Geometry: final body of the model. Coordinates: model frame, mm. Face numbers are marked on the shaded views. Give positions to 0.01 mm unless a question says otherwise; leave off trailing zeros. Order: outer loops, then holes, each group sorted by start corner. A loop starts at its lowest first (then second) coordinate and runs counter-clockwise, first axis right, second up. Notation, with made-up numbers: (-17.5, 18.25) -> (-10.5, 18.25) arc R11 cw to (-10.5, 31.25) -> close; hole circle Ø1 at (11.5, -22). An arc over 180 degrees is marked (long way). Answer in a Markdown table with one row per item. Add a question column.
Q1. Cut plane D-D on x = 12. Return the cut outline in (y, z).
Q2. Line query: line 1 along X through (y, z) = (2, 1.75); line 2 along X through (y, z) = (1, 0.5); line 3 along Z through (x, y) = (9, 6.5). Output: solid intervals per line, ascending. Write a range as from..to.
Q3. Cut plane B-B on y = 23. Return the cut outline in (x, z).
Q4. Cut plane A-A on z = 3.75. Return the cut outline in (x, y).
Q5. Contact query for flat-ended pins moving along their axis: P1, Ø3, axis at y = 3, z = 5.5, coming from the -X side; P2, Ø1.5, axis at x = 12, y = 29.5, coming from the -Z side. Output: stop coordinate, or through.
Q6. Cut plane C-C on x = 21. Return the cut outline in (y, z), and give its area (3 significant figures).
Q7. Pull-direction query (X, two-part tool) for the marked faces 1, 2, 3 and 4; classes: +X half, -X half, draft (parallel to the pull), parting line (faces both ways), or undercut.
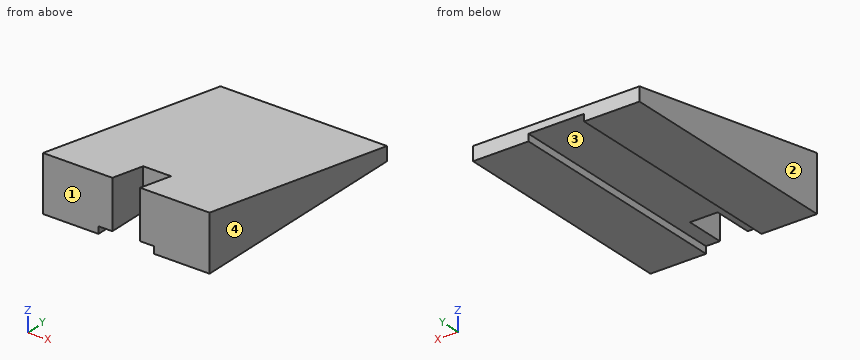
Autodesk Fusion 360 part; units mm, degrees
sketch "Sketch1" plane through (0, 0, 0) normal (0, 0, 1) x (1, 0, 0)
  line L0 (0, 0) -> (24, 0)
  line L1 (24, 0) -> (24, 34)
  line L2 (24, 34) -> (0, 34)
  line L3 (0, 34) -> (0, 0)
  line L4 (8, 34) -> (8, 0)
  line L5 (16, 34) -> (16, 0)
  dimension "d3" = 34
  dimension "d4" = 24
  dimension "d5" = 8
  dimension "d6" = 8
extrude "Extrude1" add sketch "Sketch1" along normal blind 1 contours L0 L2 L3 L4 | L0 L1 L2 L5 makes body 1 at (2.6667, 22.6667, 0) makes body 2 at (18.6667, 22.6667, 0)
sketch "Sketch2" plane through (0, 0, 0) normal (-1, 0, 0) x (0, -1, 0)
  line L0 (-34, 0) -> (0, 0)
  line L1 (0, 0) -> (0, 1)
  line L2 (0, 1) -> (-34, 1)
  line L3 (-34, 1) -> (-34, 0)
  line L4 (0, 1) -> (0, 8)
  line L5 (-34, 1) -> (-34, 2)
  line L6 (0, 8) -> (-34, 2)
  dimension "d9" = 7
  dimension "d12" = 1
extrude "Extrude3" add sketch "Sketch2" against normal up to surface (24 mm away) contours L2 L4 L5 L6 bodies 1 2
sketch "Sketch3" plane through (0, 1.3691, 7.7584) normal (0, 0.1738, 0.9848) x (-1, 0, 0)
  line L0 (-24, 1.3903) -> (-24, -33.1351)
  line L1 (-24, -33.1351) -> (0, -33.1351)
  line L2 (0, -33.1351) -> (0, 1.3903)
  line L3 (0, 1.3903) -> (-24, 1.3903)
  line L4 (-10, 1.3903) -> (-14, 1.3903)
  line L5 (-14, 1.3903) -> (-14, -4.6097)
  line L6 (-14, -4.6097) -> (-10, -4.6097)
  line L7 (-10, -4.6097) -> (-10, 1.3903)
  dimension "d15" = 4
  dimension "d16" = 6
extrude "Extrude4" cut sketch "Sketch3" along direction (0, 0.029399, 0.999568) up to surface contours L3 L4 L5 L6 L7 end surface through (0, 0, 1) normal (0, 0, -1) offset 0 bodies 1
equation "Hoogte_SERVO = 34 mm"
equation "Breedte_SERVO = 24 mm"
equation "d3 = Hoogte_SERVO"
equation "d4 = Breedte_SERVO"
equation "d6 = d5"
equation "d9 = 4 mm + 3 mm"
Completed:
| question | item | result |
|---|---|---|
| 1 | outline | (5.73, 1) -> (34, 1) -> (34, 2) -> (5.91, 6.96) -> close |
| 2 | line 1 | x = 0..10, 14..24 |
| 2 | line 2 | x = 0..8, 16..24 |
| 2 | line 3 | z = 1..6.85 |
| 3 | outline | (0, 0) -> (8, 0) -> (8, 1) -> (16, 1) -> (16, 0) -> (24, 0) -> (24, 3.94) -> (0, 3.94) -> close |
| 4 | outline | (0, 0) -> (10, 0) -> (10, 5.81) -> (14, 5.81) -> (14, 0) -> (24, 0) -> (24, 24.08) -> (0, 24.08) -> close |
| 5 | P1 | stops at x = 0 |
| 5 | P2 | stops at z = 1 |
| 6 | outline | (0, 0) -> (34, 0) -> (34, 2) -> (0, 8) -> close |
| 6 | area | 170 mm² |
| 7 | face 1 | draft |
| 7 | face 2 | -X half |
| 7 | face 3 | undercut |
| 7 | face 4 | +X half |
